```python
from build123d import *

# Parameters (mm, degrees)
SKETCH1_W           = 225
SKETCH1_H           = 225
SKETCH1_W_2         = 205
SKETCH1_H_2         = 205
WALLS_DEPTH         = 160
SKETCH1_5_W         = 205
SKETCH1_5_H         = 205
BOSS_EXTRUDE2_DEPTH = 7
SKETCH2_R           = 35.75
CUT_EXTRUDE1_DEPTH  = 197
BOSS_EXTRUDE3_START = 14
SKETCH6_R           = 50
SKETCH6_R_2         = 35.75
BOSS_EXTRUDE3_DEPTH = 14
BOSS_EXTRUDE4_START = 10
SKETCH7_R           = 50
SKETCH7_R_2         = 35.75
BOSS_EXTRUDE4_DEPTH = 10
SKETCH9_W           = 205
SKETCH9_H           = 205
CUT_EXTRUDE4_DEPTH  = 10
SKETCH10_R          = 15.75
CUT_EXTRUDE6_DEPTH  = 10
SKETCH11_R          = 15.75
CUT_EXTRUDE7_DEPTH  = 10


with BuildPart() as part:
    # Sketch1 → Walls (new body)
    with BuildSketch(Plane(origin=(0, 0, 0), x_dir=(1, 0, 0), z_dir=(0, 1, 0))):
        with Locations((-22.5, -12.5)):
            Rectangle(SKETCH1_W, SKETCH1_H)
        with Locations((-22.5, -12.5)):
            Rectangle(SKETCH1_W_2, SKETCH1_H_2, mode=Mode.SUBTRACT)
    extrude(amount=WALLS_DEPTH)

    # Sketch1_5 → Boss-Extrude2 (add)
    with BuildSketch(Plane(origin=(0, 0, 0), x_dir=(1, 0, 0), z_dir=(0, 1, 0))):
        with Locations((-22.5, -12.5)):
            Rectangle(SKETCH1_5_W, SKETCH1_5_H)
    extrude(amount=BOSS_EXTRUDE2_DEPTH)

    # Sketch2 → Cut-Extrude1 (cut)
    with BuildSketch(Plane(origin=(0, 0, -100), x_dir=(-1, 0, 0), z_dir=(0, 0, -1))):
        with Locations((22.5, 70)):
            Circle(SKETCH2_R)
    extrude(amount=-CUT_EXTRUDE1_DEPTH, mode=Mode.SUBTRACT)

    # Sketch6 → Boss-Extrude3 (add)
    with BuildSketch(Plane(origin=(0, 0, 115), x_dir=(-1, 0, 0), z_dir=(0, 0, -1)).offset(BOSS_EXTRUDE3_START)):
        with Locations(Location((22.5, 70, 0), (0, 0, 180))):
            Circle(SKETCH6_R)
        with Locations((22.5, 70)):
            Circle(SKETCH6_R_2, mode=Mode.SUBTRACT)
    extrude(amount=-BOSS_EXTRUDE3_DEPTH)

    # Sketch7 → Boss-Extrude4 (add)
    with BuildSketch(Plane(origin=(0, 0, -100), x_dir=(-1, 0, 0), z_dir=(0, 0, -1)).offset(BOSS_EXTRUDE4_START)):
        with Locations(Location((22.5, 70, 0), (0, 0, 180))):
            Circle(SKETCH7_R)
        with Locations((22.5, 70)):
            Circle(SKETCH7_R_2, mode=Mode.SUBTRACT)
    extrude(amount=-BOSS_EXTRUDE4_DEPTH)

    # Sketch9 → Cut-Extrude4 (cut)
    with BuildSketch(Plane(origin=(0, 7, 0), x_dir=(1, 0, 0), z_dir=(0, 1, 0))):
        with Locations((-22.5, -12.5)):
            Rectangle(SKETCH9_W, SKETCH9_H)
    extrude(amount=-CUT_EXTRUDE4_DEPTH, mode=Mode.SUBTRACT)

    # Sketch10 → Cut-Extrude6 (cut)
    with BuildSketch(Plane.ZY.offset(135)):
        with Locations((75, 119.5)):
            Circle(SKETCH10_R)
    extrude(amount=-CUT_EXTRUDE6_DEPTH, mode=Mode.SUBTRACT)

    # Sketch11 → Cut-Extrude7 (cut)
    with BuildSketch(Plane(origin=(90, 0, 0), x_dir=(0, 0, -1), z_dir=(1, 0, 0))):
        with Locations((50, 119.5)):
            Circle(SKETCH11_R)
    extrude(amount=-CUT_EXTRUDE7_DEPTH, mode=Mode.SUBTRACT)


solid = part.part
```
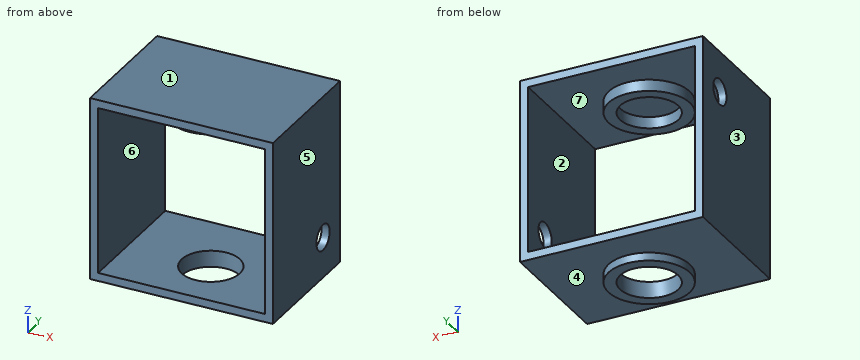
CAD build for the part. Positions are in the model's coordinates, mm. Face numbers are marked on the shaded views. A direction names the side the tool comes from. Coordinates: 2 decimals unless noted, no trailing zeros. Order: outer loops, then holes, each group sorted by start corner. A loop starts at its lowest first (then second) coordinate and runs counter-clockwise, first axis right, second up. Notation, with made-up numbers: (82.5, 79) - (131.5, 79) arc R8 ccw to (131.5, 89) - close; hole circle Ø4 at (53.5, 85). An arc over 180 degrees is marked (long way). Use a Markdown table: item, result. Add a question column.
(1) Saw through at B-B (z = -4.5). Give the cut face in (x, y), then the cut area to 3 significant figures.
(2) Saw through at D-D (x = 65). Give the cut face in (y, z), then the cut area to 3 significant figures.
(3) Drill centre lines: line 1 along Z through (x, y) = (-82.5, 138); line 2 along Y through (x, z) = (-22.5, -96.25); line 3 along X through (y, z) = (101.5, -50). Where is each one in solid material? Low to high. Write a range as [from, to].
(4) Flat gauge pins, fed straight in: pin 1 (5 mm diameter, centred on x = -97.5, y = 126.5, fed in from -Z); pin 2 (19 mm diameter, centred on y = 119.5, z = 75, fed in from -X). Where does each tip first touch, or does it go through?
(5) Which spindle directions (+Z, -Z, +X, -X, +Y, -Y) get a long thin tool onto all of the face, cutting with end or side? Do the marked faces 4, 5, 6 and 7. Say none if no direction does.
(6) Pull direction X, two halves, no side cores. Call the marked faces 1, 2 and 3: +X half, -X half, draft (parallel to the pull), parting line (faces both ways), or undercut.
(7) Saw through at C-C (z = 75). Give the cut face in (x, y), then the cut area to 4 significant figures.
(8) Saw through at A-A (x = -22.5). Give the cut face in (y, z), then the cut area to 3 significant figures.
Solved:
| question | item | result |
|---|---|---|
| 1 | outline | (-135, 0) - (-125, 0) - (-125, 160) - (-135, 160) - close; (80, 0) - (90, 0) - (90, 160) - (80, 160) - close |
| 1 | area | 3,200 mm² |
| 2 | outline | (0, -100) - (160, -100) - (160, -90) - (0, -90) - close; (0, 115) - (160, 115) - (160, 125) - (0, 125) - close |
| 2 | area | 3,200 mm² |
| 3 | line 1 | z = [-100, -90], [115, 125] |
| 3 | line 2 | y = [0, 34.25], [105.75, 160] |
| 3 | line 3 | x = [-135, -125], [80, 90] |
| 4 | pin 1 | stops at z = -100 |
| 4 | pin 2 | stops at x = 80 |
| 5 | face 4 | -Z |
| 5 | face 5 | +Z, -Z, +X, +Y, -Y |
| 5 | face 6 | +Y, -Y |
| 5 | face 7 | none |
| 6 | face 1 | draft |
| 6 | face 2 | undercut |
| 6 | face 3 | -X half |
| 7 | outline | (-135, 0) - (-125, 0) - (-125, 103.75) - (-135, 103.75) - close; (-135, 135.25) - (-125, 135.25) - (-125, 160) - (-135, 160) - close; (80, 0) - (90, 0) - (90, 160) - (80, 160) - close |
| 7 | area | 2,885 mm² |
| 8 | outline | (0, -100) - (20, -100) - (20, -110) - (34.25, -110) - (34.25, -90) - (0, -90) - close; (0, 115) - (20, 115) - (20, 101) - (34.25, 101) - (34.25, 115) - (105.75, 115) - (105.75, 101) - (120, 101) - (120, 115) - (160, 115) - (160, 125) - (0, 125) - close; (105.75, -110) - (120, -110) - (120, -100) - (160, -100) - (160, -90) - (105.75, -90) - close |
| 8 | area | 3,170 mm² |
